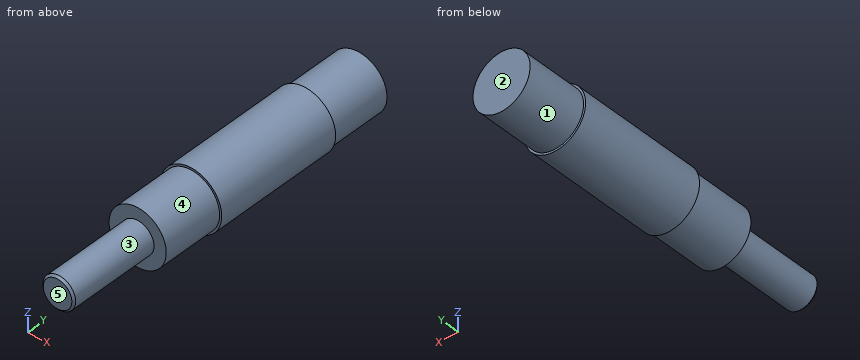
from build123d import *

# Parameters (mm, degrees)
SKETCH1_R           = 7.5
BOSS_EXTRUDE1_DEPTH = 32
SKETCH2_R           = 7
BOSS_EXTRUDE2_DEPTH = 15
BOSS_EXTRUDE3_START = 15
SKETCH3_R           = 7
BOSS_EXTRUDE3_DEPTH = 15
SKETCH4_R           = 4
BOSS_EXTRUDE4_DEPTH = 22.5
CHAMFER1_SIZE       = 0.5


with BuildPart() as part:
    # Sketch1 → Boss-Extrude1 (new body)
    with BuildSketch(Plane(origin=(0, 0, 0), x_dir=(1, 0, 0), z_dir=(0, 1, 0))):
        with Locations(Location((0, 0, 0), (0, 0, 270))):
            Circle(SKETCH1_R)
    extrude(amount=BOSS_EXTRUDE1_DEPTH)

    # Sketch2 → Boss-Extrude2 (add)
    with BuildSketch(Plane(origin=(0, 32, 0), x_dir=(1, 0, 0), z_dir=(0, 1, 0))):
        with Locations(Location((0, 0, 0), (0, 0, 270))):
            Circle(SKETCH2_R)
    extrude(amount=BOSS_EXTRUDE2_DEPTH)

    # Sketch3 → Boss-Extrude3 (add)
    with BuildSketch(Plane.XZ.offset(BOSS_EXTRUDE3_START)):
        with Locations(Location((0, 0, 0), (0, 0, 90))):
            Circle(SKETCH3_R)
    extrude(amount=-BOSS_EXTRUDE3_DEPTH)

    # Sketch4 → Boss-Extrude4 (add)
    with BuildSketch(Plane.XZ.offset(15)):
        with Locations(Location((0, 0, 0), (0, 0, 90))):
            Circle(SKETCH4_R)
    extrude(amount=BOSS_EXTRUDE4_DEPTH)

    # Chamfer1
    chamfer1_edges = [part.edges().sort_by_distance(p)[0] for p in [
        (0, -37.5, -4),
    ]]
    chamfer(chamfer1_edges, length=CHAMFER1_SIZE)


solid = part.part
Here's how the part is built. I have some questions about the finished solid (model axes, mm). Face numbers are marked on the shaded views. A direction names the side the tool comes from. Coordinates: 2 decimals unless noted, no trailing zeros. Order: outer loops, then holes, each group sorted by start corner. A loop starts at its lowest first (then second) coordinate and runs counter-clockwise, first axis right, second up. Notation, with made-up numbers: (21.5, 20) - (79.5, 20) arc R7 ccw to (79.5, 26) - close; hole circle Ø5 at (20, 66.5). An arc over 180 degrees is marked (long way). Use CSV: the item, a comma, the result in double quotes. Start each with the question number.
1. If we mould it in two halves opening along Z, with no side actions, what happens to the marked faces 4 and 5? For each: +Z half, -Z half, draft (parallel to the pull), parting line (faces both ways), or undercut.
2. For the marked faces 1, 2 and 3, which set-ups out of +Z, -Z, +X, -X, +Y, -Y let a thin tool reach every point of the face, with its end or its side?
3. Suppose I cut it at A-A on x = 0. List the corners of the cut face in (y, z) for me, then the cut area to 3 significant figures.
4. Suppose I cut it at B-B on z = 0. List the corners of the cut face in (x, y) for me, then the cut area to 3 significant figures.
5. Suppose I cut it at D-D on y = -8.5. List the corners of the cut face in (x, z) for me.
6. I'm going to push a flat-ended pin straight in: pin 1 (3 mm diameter, centred on y = -11.5, z = -2.5, fed in from -X). Where does the tip first touch, or does it pass through?
7. Suppose I cut it at C-C on y = 3.5. List the corners of the cut face in (x, z) for me.
8. Please list where these lines run through material, in increasing order: line 1 (Y direction, x = -3.25, z = 2.75); line 2 (Z direction, x = -5.75, y = 33); line 3 (Z direction, x = 0.5, y = 21). Write a range as from..to.
Output:
1,face 4,"parting line"
1,face 5,"draft"
2,face 1,"+Y"
2,face 2,"+Z, -Z, +X, -X, +Y"
2,face 3,"-Y"
3,outline,"(-37.5, -3.5) - (-37, -4) - (-15, -4) - (-15, -7) - (0, -7) - (0, -7.5) - (32, -7.5) - (32, -7) - (47, -7) - (47, 7) - (32, 7) - (32, 7.5) - (0, 7.5) - (0, 7) - (-15, 7) - (-15, 4) - (-37, 4) - (-37.5, 3.5) - close"
3,area,"1,080 mm2"
4,outline,"(-7.5, 0) - (-7, 0) - (-7, -15) - (-4, -15) - (-4, -37) - (-3.5, -37.5) - (3.5, -37.5) - (4, -37) - (4, -15) - (7, -15) - (7, 0) - (7.5, 0) - (7.5, 32) - (7, 32) - (7, 47) - (-7, 47) - (-7, 32) - (-7.5, 32) - close"
4,area,"1,080 mm2"
5,outline,"circle Ø14 at (0, 0)"
6,pin 1,"stops at x = -6.93"
7,outline,"circle Ø15 at (0, 0)"
8,line 1,"y = -15..47"
8,line 2,"z = -3.99..3.99"
8,line 3,"z = -7.48..7.48"
